Could you check a few things on this drawing? It's one solid part, dimensions in mm from its lowest x, y, z. Round coordinates to 2 decimals unless told otherwise and drop trailing zeros. Loops run counter-clockwise (first coordinate to the right, second up) from the corner with the lowest first, then second, coordinate; pieces in that order, holes last. Notation, with made-up numbers: (4, 17) -> (14, 17) arc R18 cw to (14, 24) -> close; hole circle Ø11 at (48, -20.75). An arc over 180 degrees is marked (long way). Put each result on its own line as item: value. Start each with the question number.
1. Imagine slicing it at C-C, the plane x = 105.5. Please give me the cut outline in (y, z).
2. Imagine slicing it at B-B, the plane z = 14.5. Please give me the cut outline in (x, y) (1 decimal), and give its area (3 significant figures).
3. I'm going to push flat-ended pins straight in: P1, Ø2, axis at x = 38, z = 35, coming from the -Y side; P2, Ø6, axis at y = 9, z = 43, coming from the +X side. Where does each tip first touch, or does it pass through?
4. If we mould it in two halves opening along Z, with no side actions, what happens to the marked faces 1, 2, 3 and 4? For each: pulls with the +Z half, pulls with the -Z half, needs draft (parallel to the pull), parting line crosses it, or undercut.
5. I need wall thicknesses on line 1 (X direction, y = 16, z = 30); line 2 (X direction, y = 8.25, z = 44); line 3 (Z direction, x = 126.5, y = 11). Which ranges of each line are inside material? Lowest first, please. Write a range as [from, to].
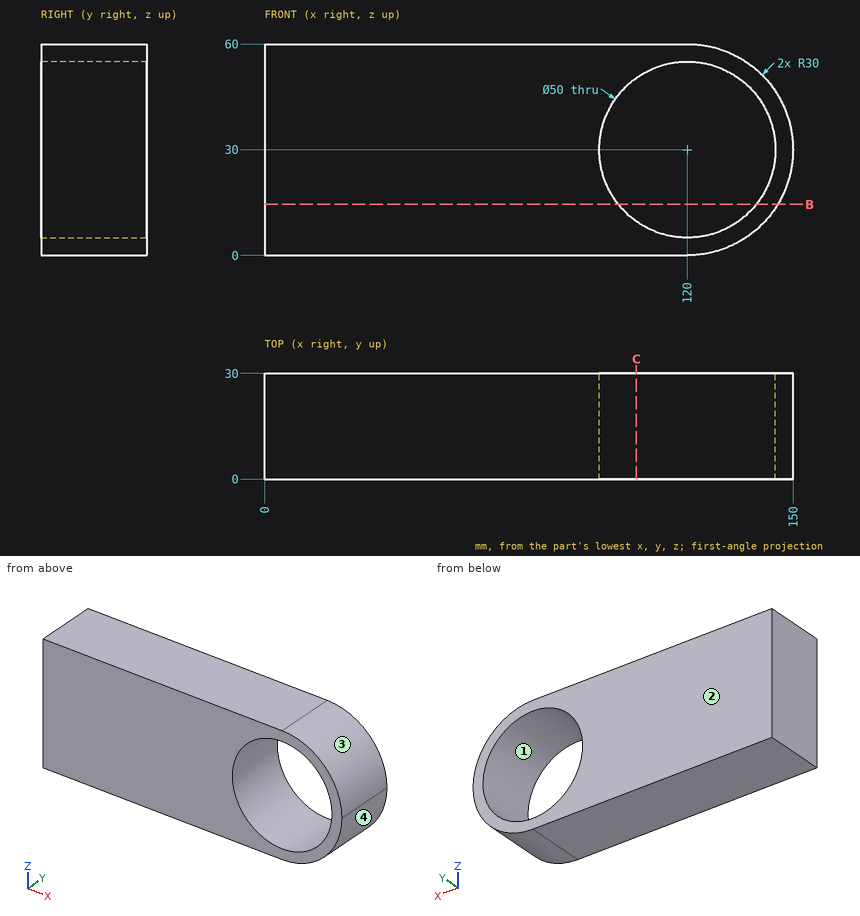
Entries:
1. outline: (0, 0) -> (30, 0) -> (30, 9.63) -> (0, 9.63) -> close; (0, 50.37) -> (30, 50.37) -> (30, 60) -> (0, 60) -> close
2. outline: (0, 0) -> (100.4, 0) -> (100.4, 30) -> (0, 30) -> close; (139.6, 0) -> (145.7, 0) -> (145.7, 30) -> (139.6, 30) -> close
2. area: 3,190 mm^2
3. P1: y = 0
3. P2: x = 148.28
4. face 1: undercut
4. face 2: needs draft
4. face 3: pulls with the +Z half
4. face 4: pulls with the -Z half
5. line 1: [0, 95], [145, 150]
5. line 2: [0, 99.29], [140.71, 146.53]
5. line 3: [0.71, 5.86], [54.14, 59.29]
